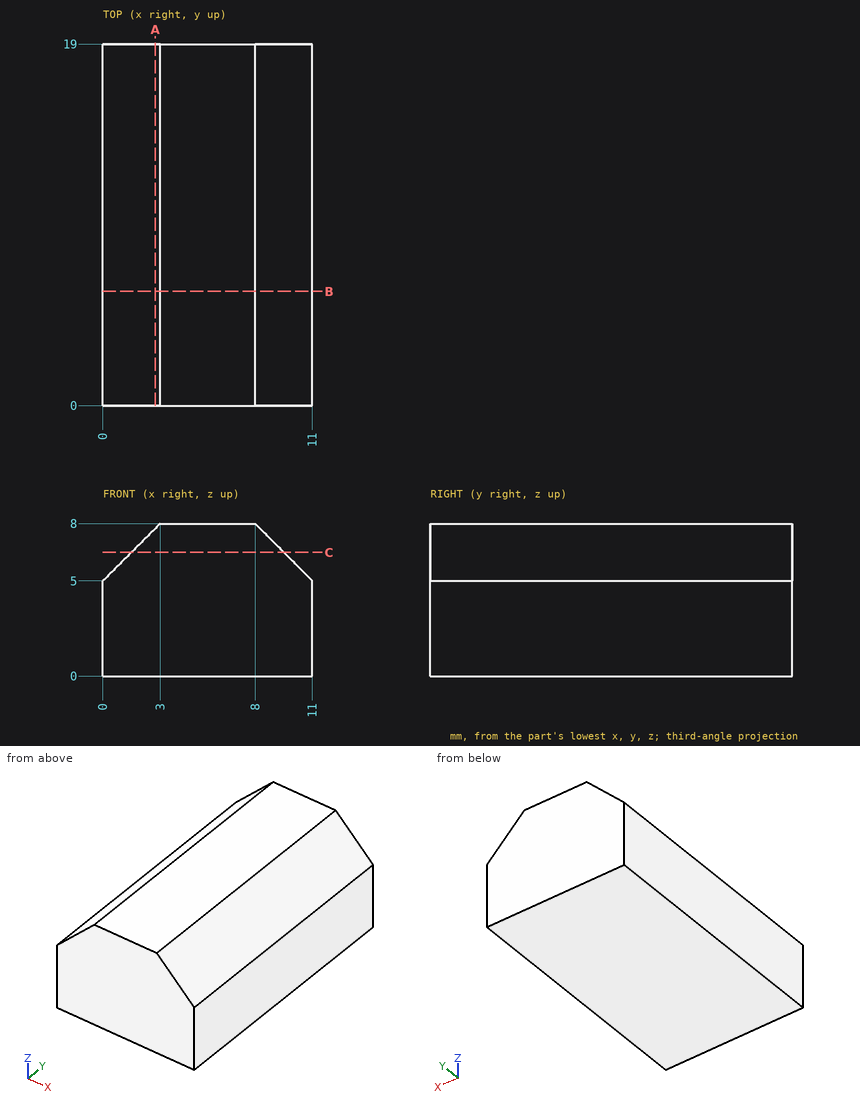
Geometry: see drawing. Coordinates: mm, zero at the bounding-box minimum. Round coordinates to 2 decimals unless told otherwise and drop trailing zeros. Loops run counter-clockwise (first coordinate to the right, second up) from the corner with the lowest first, then second, coordinate; pieces in that order, holes last.
(1) Section query A-A (x = 2.75). Output: boundary loops of the cut face in (y, z).
From the geometry:
outline: (0, 0) - (19, 0) - (19, 7.75) - (0, 7.75) - close
(2) Material intervals for probe 1 along X at (y, z) = (16, 7); probe 2 along X at (y, z) = (2, 7.25); probe 3 along Z at (x, y) = (2.75, 3), sorted ascending.
From the geometry:
probe 1: x = 2 to 9
probe 2: x = 2.25 to 8.75
probe 3: z = 0 to 7.75
(3) Section query B-B (y = 6). Output: boundary loops of the cut face in (x, z), and give its area (3 significant figures).
From the geometry:
outline: (0, 0) - (11, 0) - (11, 5) - (8, 8) - (3, 8) - (0, 5) - close
area: 79.0 mm2
(4) Section query C-C (z = 6.5). Output: boundary loops of the cut face in (x, y).
From the geometry:
outline: (1.5, 0) - (9.5, 0) - (9.5, 19) - (1.5, 19) - close
